Autodesk Inventor part; units mm, degrees
ref_plane "YZ Plane" through (0, 0, 0) normal (1, 0, 0) x (0, 1, 0)
ref_plane "XZ Plane" through (0, 0, 0) normal (0, 1, 0) x (-1, 0, 0)
ref_plane "XY Plane" through (0, 0, 0) normal (0, 0, 1) x (1, 0, 0)
sketch "スケッチ1" plane through (0, 0, 0) normal (0, 0, 1) x (1, 0, 0)
  line L0 (-2.75, 1.5877) -> (0, 3.1754)
  line L1 (0, 3.1754) -> (2.75, 1.5877)
  line L2 (2.75, 1.5877) -> (2.75, -1.5877)
  line L3 (2.75, -1.5877) -> (0, -3.1754)
  line L4 (0, -3.1754) -> (-2.75, -1.5877)
  line L5 (-2.75, -1.5877) -> (-2.75, 1.5877)
  circle A0 centre (0, 0) radius 1.5
  dimension "d0" = 5.5
  dimension "d1" = 3
extrude "押し出し1" add sketch "スケッチ1" along normal blind 8 contours L0 L1 L2 L3 L4 L5 | A0
sketch "スケッチ2" plane through (0, 0, 8) normal (0, 0, 1) x (1, 0, 0)
  circle A0 centre (0, 0) radius 1.5
  dimension "d4" = 3
extrude "押し出し2" add sketch "スケッチ2" along normal blind 6
extrude "押し出し3" add sketch "スケッチ1" against normal blind 6 contours A0
properties part number "スペーサー　両雄ねじ　m3-8" material "アルミニウム 2014-T4"
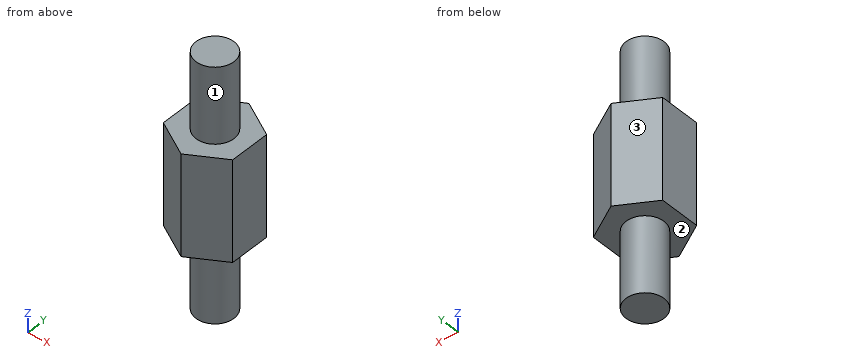
Input: part model. Units: mm. Frame: model coordinates. Face numbers are marked on the shaded views. A direction names the side the tool comes from. Round coordinates to 2 decimals unless told otherwise and drop trailing zeros. Loops run counter-clockwise (first coordinate to the right, second up) from the corner with the lowest first, then second, coordinate; pieces in that order, holes last. Notation, with made-up numbers: M -17,82.5 L 33,82.5 A26 cw 33,114.5 Z; hole C 2,44.5 d3. An arc over 180 degrees is marked long. Answer in a Markdown table with one row per item. Add a question column.
1. Set-up query: the marked faces 1, 2 and 3. Return all of +Z, -Z, +X, -X, +Y, -Y with unobstructed straight access to the full face (end or side cutting, diameter ignored); none if empty.
2. Section A-A (y = 0). Output: boundary loops of the cut face in (x, z).
3. Section C-C (x = -0.55). Output: boundary loops of the cut face in (y, z).
4. Section B-B (z = 0.5). Output: boundary loops of the cut face in (x, y), and give its area (3 significant figures).
5. Ray query, probe 1 along Z at (x, y) = (1.5, -1.75); probe 2 along Y at (x, z) = (0, 9.25); probe 3 along X at (y, z) = (1.25, 10.75). Return the intervals inside material, ascending.
6. Section D-D (z = -3.75). Output: boundary loops of the cut face in (x, y), and give its area (3 significant figures).
Values follow:
| question | item | result |
|---|---|---|
| 1 | face 1 | +Z |
| 1 | face 2 | -Z |
| 1 | face 3 | +Z, -Z, -X, +Y |
| 2 | outline | M -2.75,0 L -1.5,0 L -1.5,-6 L 1.5,-6 L 1.5,0 L 2.75,0 L 2.75,8 L 1.5,8 L 1.5,14 L -1.5,14 L -1.5,8 L -2.75,8 Z |
| 3 | outline | M -2.86,0 L -1.4,0 L -1.4,-6 L 1.4,-6 L 1.4,0 L 2.86,0 L 2.86,8 L 1.4,8 L 1.4,14 L -1.4,14 L -1.4,8 L -2.86,8 Z |
| 4 | outline | M -2.75,-1.59 L 0,-3.18 L 2.75,-1.59 L 2.75,1.59 L 0,3.18 L -2.75,1.59 Z |
| 4 | area | 26.2 mm^2 |
| 5 | probe 1 | 0 to 8 |
| 5 | probe 2 | -1.5 to 1.5 |
| 5 | probe 3 | -0.83 to 0.83 |
| 6 | outline | C 0,0 d3 |
| 6 | area | 7.07 mm^2 |
